Print and shaded views of the part. All mm, measured from the part's lowest x, y and z. Round coordinates to 2 decimals unless told otherwise and drop trailing zeros. Write each loop counter-clockwise with the first axis right and the second up, starting at its lowest first coordinate (ties: lowest second). Pieces come first, ordered by that corner, then holes. Notation, with made-up numbers: (27, -37) - (48, -37) arc R26 ccw to (48, -10) - close; hole circle Ø8 at (37.5, 66). An arc over 180 degrees is marked (long way). One line per item, written item: value.
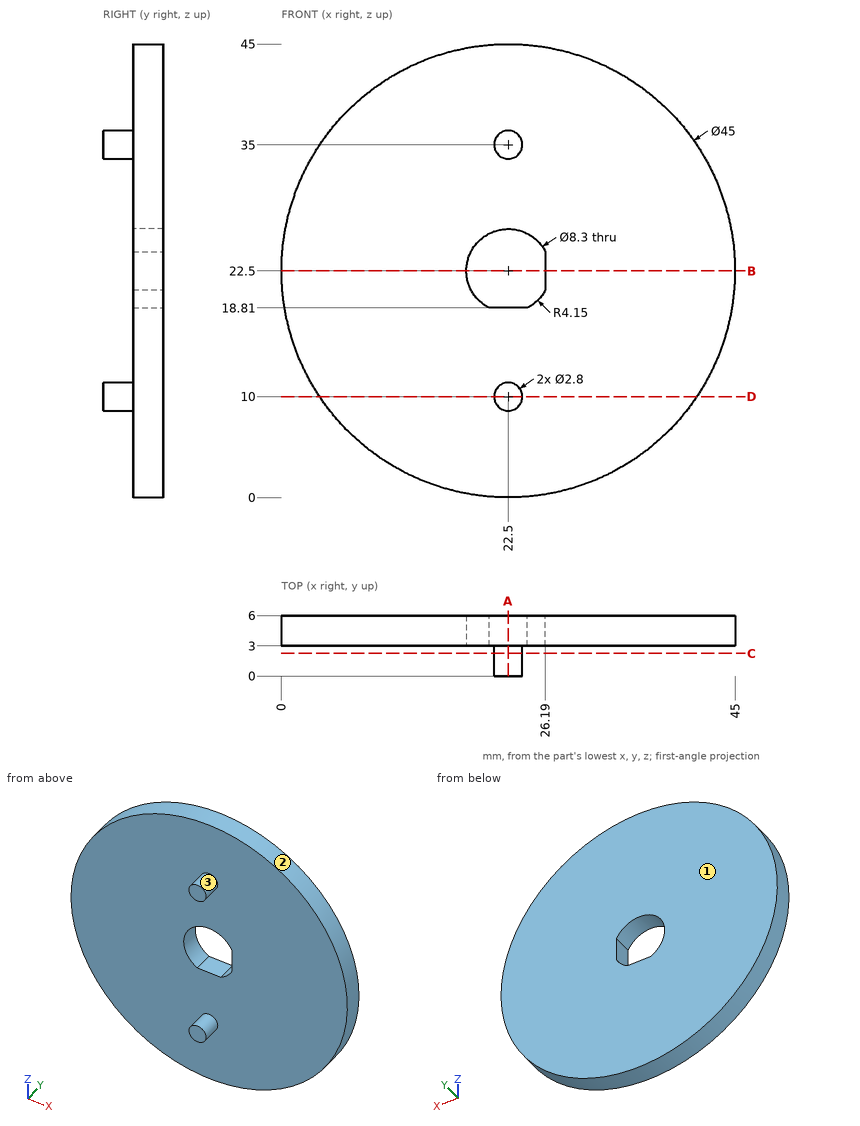
1. Wall check: probe 1 along X at (y, z) = (4.4, 22.5); probe 2 along Y at (x, z) = (8.5, 26); probe 3 along X at (y, z) = (0.65, 10). Give the ranges that are in metal, low to high. Write a range as [from, to].
Report:
probe 1: [0, 18.35], [26.19, 45]
probe 2: [3, 6]
probe 3: [21.1, 23.9]
2. Band-saw the part on B-B on z = 22.5. Write the cut outline in (x, y).
Report:
outline: (0, 3) - (18.35, 3) - (18.35, 6) - (0, 6) - close; (26.19, 3) - (45, 3) - (45, 6) - (26.19, 6) - close
3. Mould opens along Z. For the marked faces 1, 2 and 3 say: released by +Z, released by -Z, zero draft, split by the parting line, or undercut.
Report:
face 1: zero draft
face 2: split by the parting line
face 3: undercut
4. Band-saw the part on D-D on z = 10. Write the cut outline in (x, y).
Report:
outline: (3.79, 3) - (21.1, 3) - (21.1, 0) - (23.9, 0) - (23.9, 3) - (41.21, 3) - (41.21, 6) - (3.79, 6) - close
5. Drop flat-ended pins along their axis: pin 1 (2 mm diameter, centred on y = 2.5, z = 14, fed in from +X) (1 decimal); pin 2 (1 mm diameter, centred on y = 4, z = 9, fed in from +X) (1 decimal); pin 3 (3 mm diameter, centred on x = 20.5, z = 13, fed in from -Y); pin 4 (6.5 mm diameter, centred on x = 22.5, z = 22.5, fed in from -Y). Give the stop position or say it passes through.
Report:
pin 1: x = 43.7
pin 2: x = 40.9
pin 3: y = 3
pin 4: through
6. Band-saw the part on A-A on x = 22.5. Write the cut outline in (y, z).
Report:
outline: (0, 8.6) - (3, 8.6) - (3, 0) - (6, 0) - (6, 18.81) - (3, 18.81) - (3, 11.4) - (0, 11.4) - close; (0, 33.6) - (3, 33.6) - (3, 26.65) - (6, 26.65) - (6, 45) - (3, 45) - (3, 36.4) - (0, 36.4) - close
7. Band-saw the part on C-C on y = 2.25. Write the cut outline in (x, z).
Report:
outline: circle Ø2.8 at (22.5, 10); circle Ø2.8 at (22.5, 35)
